from build123d import *

# Parameters (mm, degrees)
BOSS_EXTRUDE1_DEPTH = 152.4


with BuildPart() as part:
    # Sketch2 → Boss-Extrude1 (new body)
    with BuildSketch(Plane(origin=(0, 0, 0), x_dir=(1, 0, 0), z_dir=(0, 1, 0))):
        Polygon((0, 57.15), (-14.212627051, 55.354527659), (-27.532222475, 50.080926765), (-39.121867104, 41.660557057), (-48.253340942, 30.622501333), (-54.352879906, 17.660321229), (-57.03722753, 3.588478191), (-56.137716379, -10.708842129), (-51.710866048, -24.333286513), (-44.034831825, -36.428781014), (-33.591927169, -46.235321229), (-21.038318186, -53.136726169), (-7.162794298, -56.69935518), (7.162794298, -56.69935518), (21.038318186, -53.136726169), (33.591927169, -46.235321229), (44.034831825, -36.428781014), (51.710866048, -24.333286513), (56.137716379, -10.708842129), (57.03722753, 3.588478191), (54.352879906, 17.660321229), (48.253340942, 30.622501333), (39.121867104, 41.660557057), (27.532222475, 50.080926765), (14.212627051, 55.354527659), align=None)
        Polygon((0, 52.07), (-12.949282425, 50.4341252), (-25.08491381, 45.62928883), (-35.644367806, 37.95739643), (-43.964155081, 27.900501215), (-49.521512803, 16.090514897), (-51.967251749, 3.269502352), (-51.147697145, -9.75694505), (-47.114344622, -22.170327712), (-40.120624551, -33.190667146), (-30.605978087, -42.125514897), (-19.168245458, -48.41346162), (-6.526101472, -51.659412497), (6.526101472, -51.659412497), (19.168245458, -48.41346162), (30.605978087, -42.125514897), (40.120624551, -33.190667146), (47.114344622, -22.170327712), (51.147697145, -9.75694505), (51.967251749, 3.269502352), (49.521512803, 16.090514897), (43.964155081, 27.900501215), (35.644367806, 37.95739643), (25.08491381, 45.62928883), (12.949282425, 50.4341252), align=None, mode=Mode.SUBTRACT)
    extrude(amount=BOSS_EXTRUDE1_DEPTH)


solid = part.part
For this review, take the finished solid that the model builds, in its own axes (mm). A direction names the side the tool comes from. Round coordinates to 2 decimals unless told otherwise and drop trailing zeros. Loops run counter-clockwise (first coordinate to the right, second up) from the corner with the lowest first, then second, coordinate; pieces in that order, holes last. Notation, with made-up numbers: (-10, -1.5) - (49, -1.5) arc R32 ccw to (49, 34.5) - close; hole circle Ø10 at (58.25, 19). An arc over 180 degrees is marked (long way). Put each result on its own line as item: value. Start each with the question number.
1. Consider section B-B on z = -48. State the section outline as (x, y) points, plus the area to 3 significant figures.
2. Consider section A-A on z = -36. State the section outline as (x, y) points.
3. Insertion check: P1, Ø5, axis at y = 114, z = -44, coming from the -X side; P2, Ø12, axis at y = 89, z = 34, coming from the -X side; P3, Ø10.5, axis at x = -2.5, y = 79, coming from the -Z side; P4, Ø1, axis at x = -45, z = 25, coming from the -Y side. Each pin has a flat end and moves straight along its axis. Give the tip position at first contact, or say it passes through.
4. For probe 1 along X at (y, z) = (118.5, 17); probe 2 along Z at (x, y) = (-14, 38); probe 3 along X at (y, z) = (83, 28.5), list the stretches that pass through material, from the lowest coordinate up. Write a range as [from, to].
5. Mouldability with a two-part tool opening along Z and no side actions: class faces 1 (the flat face through (-38.89, 75.13, 41.26)), 2 (the flat face through (49.103, 75.133, 16.051)), 3 (the flat face through (-7.007, 75.133, -56.265)) as +Z half, -Z half, draft (parallel to the pull), parting line (faces both ways), or undercut.
6. For faces 4 (the flat face through (-49.16, 75.13, 15.88)), 5 (the flat face through (-51.26, 75.13, -24.23)), list the 3-axis set-ups (+Z, -Z, +X, -X, +Y, -Y) from which the entire face can be reached by the end or side of a thin tool; tool diameter is ignored.
Result sheet:
1. outline: (-30.4, 0) - (-19.1, 0) - (-19.1, 152.4) - (-30.4, 152.4) - close; (19.1, 0) - (30.4, 0) - (30.4, 152.4) - (19.1, 152.4) - close
1. area: 3,440 mm^2
2. outline: (-43.8, 0) - (-37.26, 0) - (-37.26, 152.4) - (-43.8, 152.4) - close; (37.26, 0) - (43.8, 0) - (43.8, 152.4) - (37.26, 152.4) - close
3. P1: x = -39.25
3. P2: x = -49.38
3. P3: z = -57.15
3. P4: y = 0
4. probe 1: [-54.09, -48.79], [48.79, 54.09]
4. probe 2: [-55.38, -50.02], [49.74, 54.94]
4. probe 3: [-49.07, -43.1], [43.1, 49.07]
5. face 1: +Z half
5. face 2: undercut
5. face 3: -Z half
6. face 4: +Y, -Y
6. face 5: -Z, -X, +Y, -Y
